Study the drawing (mm; zero at the part's minimum x, y, z) and answer. Give positions to 0.01 mm unless a question says otherwise; leave off trailing zeros. Loops run counter-clockwise (first coordinate to the right, second up) from the corner with the lowest first, then second, coordinate; pieces in that order, holes last. Notation, with made-up numbers: M 71.5,44.25 L 93.5,44.25 A12 ccw 93.5,62.25 Z; hole C 87,-9.5 d7. An arc over 180 degrees is marked long. Use one line per item in the form item = value. Start each with the question number.
1. The part is cut by section B-B (x = 17.5). Write down the section's boundary in (y, z).
2. The part is cut by section C-C (y = 18.5). Write down the section's boundary in (x, z).
3. The part is cut by section D-D (x = 38.5). Give the number of separate pieces and of enclosed holes in the cut face.
4. The part is cut by section A-A (y = 3). Write down the section's boundary in (x, z), and give its area (3 significant figures).
5. This flat-tipped pin is pushed along its axis until it touches: pin 1 Ø2.5 at (x, y) = (3, 57) entering from +Z. Where does it stop, or does it pass through?
6. Straight lines are drawn through the part: line 1 (X direction, y = 41, z = 0.6); line 2 (Y direction, x = 3, z = 2.2); line 3 (Y direction, x = 17.5, z = 0.9). For each, find the intervals that lie inside material, in ascending order. Write a range as from..to.
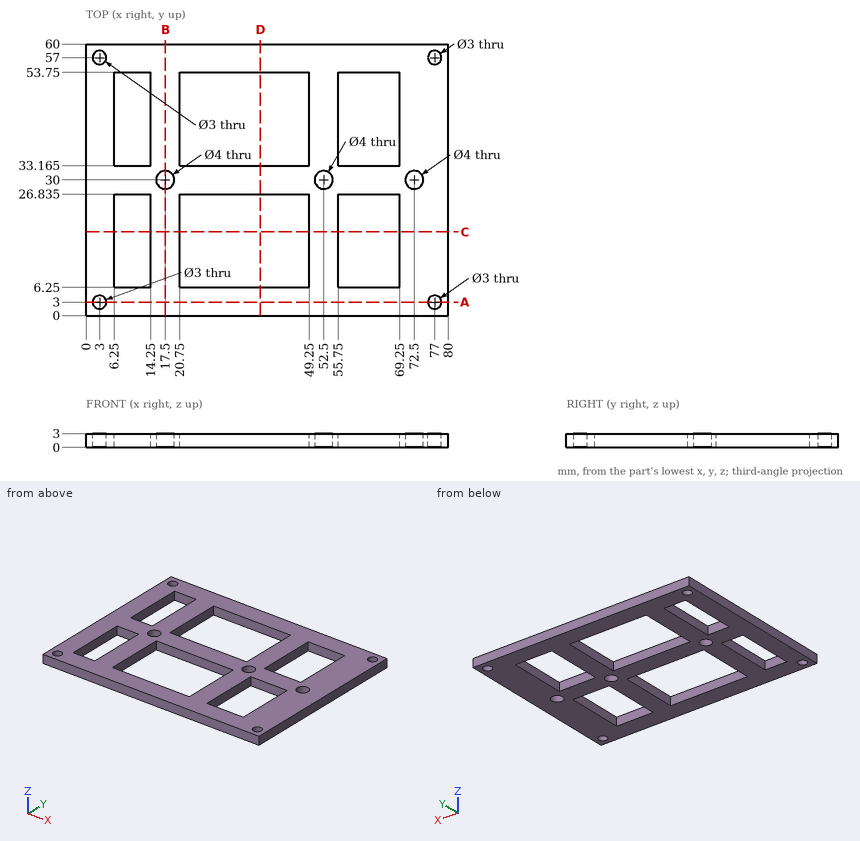
Derived:
q1.outline = M 0,0 L 28,0 L 28,3 L 0,3 Z; M 32,0 L 60,0 L 60,3 L 32,3 Z
q2.outline = M 0,0 L 6.25,0 L 6.25,3 L 0,3 Z; M 14.25,0 L 20.75,0 L 20.75,3 L 14.25,3 Z; M 49.25,0 L 55.75,0 L 55.75,3 L 49.25,3 Z; M 69.25,0 L 80,0 L 80,3 L 69.25,3 Z
q3.separate_pieces = 3
q3.enclosed_holes = 0
q4.outline = M 0,0 L 1.5,0 L 1.5,3 L 0,3 Z; M 4.5,0 L 75.5,0 L 75.5,3 L 4.5,3 Z; M 78.5,0 L 80,0 L 80,3 L 78.5,3 Z
q4.area = 222 mm2
q5.pin_1 = through
q6.line_1 = 0..6.25, 14.25..20.75, 49.25..55.75, 69.25..80
q6.line_2 = 0..1.5, 4.5..55.5, 58.5..60
q6.line_3 = 0..28, 32..60
